Source: CAD feature listing. Evaluate the final solid. Frame: model axes, mm. A direction names the side the tool comes from. Give positions to 0.01 mm unless a question says otherwise; leave off trailing zeros. Order: outer loops, then holes, each group sorted by start corner. A loop starts at its lowest first (then second) coordinate and runs counter-clockwise, first axis right, second up. Notation, with made-up numbers: M 31,6 L 80,6 A5 ccw 80,15 Z; hole C 68,-0.5 d2. An arc over 180 degrees is marked long. Return JSON: item names as keys, results as strings.
from build123d import *

# Parameters (mm, degrees)
SKETCH1_R           = 43.815
SKETCH1_R_2         = 41.275
EXTRUDE_THIN1_DEPTH = 57.15
CUT_EXTRUDE12_DEPTH = 85.29490465
CHAMFER1_SIZE       = 2.54
BOSS_EXTRUDE1_START = 2.54
BOSS_EXTRUDE1_DEPTH = 2.54


with BuildPart() as part:
    # Sketch1 → Extrude-Thin1 (new body)
    with BuildSketch(Plane(origin=(0, 0, 0), x_dir=(1, 0, 0), z_dir=(0, 1, 0))):
        Circle(SKETCH1_R)
        Circle(SKETCH1_R_2, mode=Mode.SUBTRACT)
    extrude(amount=EXTRUDE_THIN1_DEPTH)

    # Sketch4 → Cut-Extrude12 (cut, through all)
    with BuildSketch(Plane(origin=(0, 57.15, 0), x_dir=(1, 0, 0), z_dir=(0, 1, 0))):
        with BuildLine():
            Line((-41.275, 0), (-43.815, 0))
            ThreePointArc((-43.815, 0), (-37.944903067, 21.9075), (-21.9075, 37.944903067))
            Line((-21.9075, 37.944903067), (-20.6375, 35.745198541))
            ThreePointArc((-20.6375, 35.745198541), (-35.745198541, 20.6375), (-41.275, 0))
        make_face()
    extrude(amount=-CUT_EXTRUDE12_DEPTH, mode=Mode.SUBTRACT)

    # Chamfer1
    # the kernel refuses this chamfer: 5.08, 2.54 mm, written as the material it takes off along each edge
    with BuildSketch(Plane(origin=(-43.815, 69.10149318, 0), x_dir=(0.0525256370506935, 0, 0.998619575940918), z_dir=(0, -1, 0))) as chamfer1_piece_1:
        with BuildLine():
            Line((4.602821575, 0), (CHAMFER1_SIZE * 0.0525256370507, -CHAMFER1_SIZE * 0.998619575941))
            Line((CHAMFER1_SIZE * 0.0525256370507, -CHAMFER1_SIZE * 0.998619575941), (0, 0))
            ThreePointArc((0, 0), (2.389793213, 0.060394139), (4.602821575, 0))
        make_face()
    extrude(amount=81.05298636, mode=Mode.SUBTRACT)

    # Sketch5 → Boss-Extrude1 (add)
    with BuildSketch(Plane.XZ.offset(BOSS_EXTRUDE1_START)):
        with BuildLine():
            Line((-21.9075, -37.944903067), (-43.573233865, 4.596467729))
            ThreePointArc((-43.573233865, 4.596467729), (39.043228403, 19.884178154), (-21.9075, -37.944903067))
        make_face()
    extrude(amount=-BOSS_EXTRUDE1_DEPTH)


solid = part.part
1. Set-up query: faces 4 (the face through (-42.44, 28.98, 2.33)), 5 (the face through (1, 0, 1)). Return all of +Z, -Z, +X, -X, +Y, -Y with unobstructed straight access to the full face (end or side cutting, diameter ignored); none if empty.
Evaluation:
{"face 4": "-Z, -X, +Y, -Y", "face 5": "+Y"}
2. Section query A-A (x = 0). Return loops of the section in (y, z) (3 decimals), then the cut area to 3 significant figures.
Evaluation:
{"outline": "M -2.54,-43.815 L 57.15,-43.815 L 57.15,-41.275 L 0,-41.275 L 0,41.275 L 57.15,41.275 L 57.15,43.815 L -2.54,43.815 Z", "area": "513 mm^2"}
3. Ray query, probe 1 along Z at (x, y) = (0, 34.5) (3 decimals); probe 2 along Y at (x, z) = (-29, 20); probe 3 along Z at (x, y) = (3, 39). Return the intervals inside material, ascending.
Evaluation:
{"probe 1": "z = -43.815 to -41.275, 41.275 to 43.815", "probe 2": "y = -2.54 to 0", "probe 3": "z = -43.71 to -41.17, 41.17 to 43.71"}
4. First-contact query: pin 1 (8 mm diameter, centred on x = -8.5, z = -21.5, fed in from +Y); pin 2 (6 mm diameter, centred on x = -30.5, y = 19, fed in from -Z); pin 3 (5 mm diameter, centred on y = 36.5, z = 13.5, fed in from +X). Flat tips, straight axial feed; report the tip coordinate or a pass-through.
Evaluation:
{"pin 1": "stops at y = 0", "pin 2": "stops at z = 24.11", "pin 3": "stops at x = 42.41"}
5. Section query B-B (z = -2). Return loops of the section in (x, y).
Evaluation:
{"outline": "M -40.21,-2.54 L 43.77,-2.54 L 43.77,57.15 L 41.23,57.15 L 41.23,0 L -40.21,0 Z"}
6. Draft query along Z for faces 1 (the face through (-32.59, -1.29, -16.97)), 2 (the face through (39, 57.15, 16)), 3 (the face through (-21.28, 28.98, -36.86)). Return one class per face: pulls with the +Z half, pulls with the -Z half, needs draft (parallel to the pull), parting line crosses it, or undercut.
Evaluation:
{"face 1": "pulls with the -Z half", "face 2": "needs draft", "face 3": "undercut"}
7. Section query D-D (x = 18). Return loops of the section in (y, z), then the cut area to 3 significant figures.
Evaluation:
{"outline": "M -2.54,-39.95 L 57.15,-39.95 L 57.15,-37.14 L 0,-37.14 L 0,37.14 L 57.15,37.14 L 57.15,39.95 L -2.54,39.95 Z", "area": "523 mm^2"}
